The model under review builds one solid part; all positions refer to its coordinate system, in mm. A direction names the side the tool comes from. Coordinates: 2 decimals unless noted, no trailing zeros. Order: outer loops, then holes, each group sorted by start corner. A loop starts at its lowest first (then second) coordinate and runs counter-clockwise, first axis right, second up. Notation, with made-up numbers: (88, 6) - (132, 6) arc R17 cw to (132, 21) - close; hole circle Ø11 at (74.25, -11). An arc over 180 degrees is marked (long way). Answer in a Markdown table with one row per item.
```python
from build123d import *

# Parameters (mm, degrees)
SKETCH1_R           = 1.5
BOSS_EXTRUDE1_DEPTH = 3
SKETCH2_R           = 8
CUT_EXTRUDE1_DEPTH  = 0.7
SKETCH3_R           = 1.6
CUT_EXTRUDE3_DEPTH  = 10.5


with BuildPart() as part:
    # Sketch1 → Boss-Extrude1 (new body)
    with BuildSketch(Plane(origin=(0, 0, 0), x_dir=(1, 0, 0), z_dir=(0, 1, 0))):
        with BuildLine():
            Line((-14.325510257, -2.5), (14.325510257, -2.5))
            ThreePointArc((14.325510257, -2.5), (20.275, 0), (14.325510257, 2.5))
            Line((14.325510257, 2.5), (-14.325510257, 2.5))
            ThreePointArc((-14.325510257, 2.5), (-20.275, 0), (-14.325510257, -2.5))
        make_face()
        with Locations(Location((16.775, 0, 0), (0, 0, 270))):
            Circle(SKETCH1_R, mode=Mode.SUBTRACT)
        with Locations(Location((-16.775, 0, 0), (0, 0, 270))):
            Circle(SKETCH1_R, mode=Mode.SUBTRACT)
    extrude(amount=BOSS_EXTRUDE1_DEPTH)

    # Sketch2 → Cut-Extrude1 (cut)
    with BuildSketch(Plane(origin=(0, 3, 0), x_dir=(1, 0, 0), z_dir=(0, 1, 0))):
        with Locations((-16.775, 0)):
            Circle(SKETCH2_R)
        with Locations((16.775, 0)):
            Circle(SKETCH2_R)
    extrude(amount=-CUT_EXTRUDE1_DEPTH, mode=Mode.SUBTRACT)

    # Sketch3 → Cut-Extrude3 (cut)
    with BuildSketch(Plane(origin=(0, 2.3, 0), x_dir=(1, 0, 0), z_dir=(0, 1, 0))):
        with Locations(Location((-16.775, 0, 0), (0, 0, 270))):
            Circle(SKETCH3_R)
        with Locations(Location((16.775, 0, 0), (0, 0, 270))):
            Circle(SKETCH3_R)
    extrude(amount=-CUT_EXTRUDE3_DEPTH, mode=Mode.SUBTRACT)


solid = part.part
```
Item 1: Mouldability with a two-part tool opening along X and no side actions: class faces 4 (the face through (0, 0, 0)), 5 (the face through (-20.273, 1.134, -0.115)) as +X half, -X half, draft (parallel to the pull), parting line (faces both ways), or undercut.
Check values:
| item | result |
|---|---|
| face 4 | draft |
| face 5 | undercut |
Item 2: Clearance check with flat-ended pins moving along their axes: pin 1 Ø1.5 at (x, y) = (5, 2) entering from -Z; pin 2 Ø1.5 at (x, y) = (3, 2) entering from +Z; pin 3 Ø1.5 at (x, z) = (-10.5, -1.5) entering from +Y. State where each tip first meets the part, or that it passes through.
Check values:
| item | result |
|---|---|
| pin 1 | z = -2.5 |
| pin 2 | z = 2.5 |
| pin 3 | y = 2.3 |
Item 3: We need section D-D, the plane x = 13. Write out the cut boundary in (y, z).
Check values:
| item | result |
|---|---|
| outline | (0, -2.5) - (2.3, -2.5) - (2.3, 2.5) - (0, 2.5) - close |
Item 4: We need section A-A, the plane z = 0. Write out the cut boundary in (x, y) (3 decimals), then the cut area to 3 significant figures.
Check values:
| item | result |
|---|---|
| outline | (-20.275, 0) - (-18.375, 0) - (-18.375, 2.3) - (-20.275, 2.3) - close; (-15.175, 0) - (15.175, 0) - (15.175, 2.3) - (8.775, 2.3) - (8.775, 3) - (-8.775, 3) - (-8.775, 2.3) - (-15.175, 2.3) - close; (18.375, 0) - (20.275, 0) - (20.275, 2.3) - (18.375, 2.3) - close |
| area | 90.8 mm^2 |
Item 5: We need section C-C, the plane x = -1. Write out the cut boundary in (y, z), then the cut area to 3 significant figures.
Check values:
| item | result |
|---|---|
| outline | (0, -2.5) - (3, -2.5) - (3, 2.5) - (0, 2.5) - close |
| area | 15.0 mm^2 |
Item 6: Tool access review of faces 1 (the face through (0, 1, 2.5)), 2 (the face through (20.273, 1.134, 0.115)), 3 (the face through (0, 1, -2.5)): name each direction out of +Z, -Z, +X, -X, +Y, -Y from which nothing blocks a thin tool from reaching the whole face with its end or side.
Check values:
| item | result |
|---|---|
| face 1 | +Z, +Y, -Y |
| face 2 | +Y, -Y |
| face 3 | -Z, +Y, -Y |
Item 7: We need section B-B, the plane y = 0.5. Write out the cut boundary in (x, z) (3 decimals), then the cut area to 3 significant figures.
Check values:
| item | result |
|---|---|
| outline | (-14.326, -2.5) - (14.326, -2.5) arc R3.5 ccw (long way) to (14.326, 2.5) - (-14.326, 2.5) arc R3.5 ccw (long way) to start; hole circle Ø3.2 at (-16.775, 0); hole circle Ø3.2 at (16.775, 0) |
| area | 197 mm^2 |
Item 8: To check wall thickness, follow line 1 (X direction, y = 1.2, z = 0) (3 decimals); line 2 (X direction, y = 2.25, z = 0.5); line 3 (Z direction, x = -14, y = 1.75). State the ranges of each line that lie inside material, in increasing order. Write a range as from..to.
Check values:
| item | result |
|---|---|
| line 1 | -20.275..-18.375, -15.175..15.175, 18.375..20.275 |
| line 2 | -20.24..-18.29, -15.26..15.26, 18.29..20.24 |
| line 3 | -2.5..2.5 |
